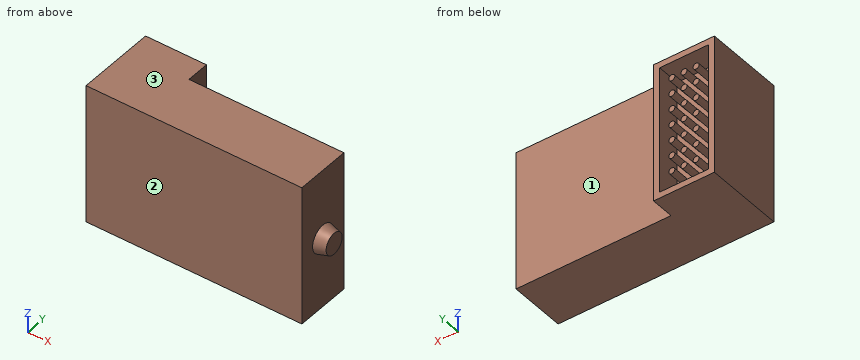
```python
from build123d import *

# Parameters (mm, degrees)
SKETCH1_W           = 35.5
SKETCH1_H           = 23
BOSS_EXTRUDE1_DEPTH = 9.18
SKETCH2_W           = 10
SKETCH2_H           = 23
SKETCH2_W_2         = 8
SKETCH2_H_2         = 21
BOSS_EXTRUDE2_DEPTH = 3.82
SKETCH3_R           = 0.5
BOSS_EXTRUDE3_DEPTH = 3.82


with BuildPart() as part:
    # Sketch1 → Boss-Extrude1 (new body)
    with BuildSketch(Plane(origin=(0, 0, 0), x_dir=(1, 0, 0), z_dir=(0, 1, 0))):
        Rectangle(SKETCH1_W, SKETCH1_H)
    extrude(amount=BOSS_EXTRUDE1_DEPTH)

    # Sketch2 → Boss-Extrude2 (add)
    with BuildSketch(Plane(origin=(0, 9.18, 0), x_dir=(1, 0, 0), z_dir=(0, 1, 0))):
        with Locations((-12.75, 0)):
            Rectangle(SKETCH2_W, SKETCH2_H)
        with Locations((-12.75, 0)):
            Rectangle(SKETCH2_W_2, SKETCH2_H_2, mode=Mode.SUBTRACT)
    extrude(amount=BOSS_EXTRUDE2_DEPTH)

    # Sketch3 → Boss-Extrude3 (add)
    with BuildSketch(Plane(origin=(0, 9.18, 0), x_dir=(1, 0, 0), z_dir=(0, 1, 0))):
        with Locations(Location((-14.75, 7.875, 0), (0, 0, 90))):
            Circle(SKETCH3_R)
        with Locations(Location((-12.75, 7.875, 0), (0, 0, 90))):
            Circle(SKETCH3_R)
        with Locations(Location((-10.75, 7.875, 0), (0, 0, 90))):
            Circle(SKETCH3_R)
        with Locations(Location((-12.75, 5.25, 0), (0, 0, 90))):
            Circle(SKETCH3_R)
        with Locations(Location((-10.75, 5.25, 0), (0, 0, 90))):
            Circle(SKETCH3_R)
        with Locations(Location((-12.75, 2.625, 0), (0, 0, 90))):
            Circle(SKETCH3_R)
        with Locations(Location((-10.75, 2.625, 0), (0, 0, 90))):
            Circle(SKETCH3_R)
        with Locations(Location((-12.75, 0, 0), (0, 0, 90))):
            Circle(SKETCH3_R)
        with Locations(Location((-10.75, 0, 0), (0, 0, 90))):
            Circle(SKETCH3_R)
        with Locations(Location((-12.75, -2.625, 0), (0, 0, 90))):
            Circle(SKETCH3_R)
        with Locations(Location((-10.75, -2.625, 0), (0, 0, 90))):
            Circle(SKETCH3_R)
        with Locations(Location((-12.75, -5.25, 0), (0, 0, 90))):
            Circle(SKETCH3_R)
        with Locations(Location((-10.75, -5.25, 0), (0, 0, 90))):
            Circle(SKETCH3_R)
        with Locations(Location((-12.75, -7.875, 0), (0, 0, 90))):
            Circle(SKETCH3_R)
        with Locations(Location((-10.75, -7.875, 0), (0, 0, 90))):
            Circle(SKETCH3_R)
        with Locations(Location((-14.75, 5.25, 0), (0, 0, 90))):
            Circle(SKETCH3_R)
        with Locations(Location((-14.75, 2.625, 0), (0, 0, 90))):
            Circle(SKETCH3_R)
        with Locations(Location((-14.75, 0, 0), (0, 0, 90))):
            Circle(SKETCH3_R)
        with Locations(Location((-14.75, -2.625, 0), (0, 0, 90))):
            Circle(SKETCH3_R)
        with Locations(Location((-14.75, -5.25, 0), (0, 0, 90))):
            Circle(SKETCH3_R)
        with Locations(Location((-14.75, -7.875, 0), (0, 0, 90))):
            Circle(SKETCH3_R)
    extrude(amount=BOSS_EXTRUDE3_DEPTH)

    # Sketch5 → Revolve1 (revolve)
    with BuildSketch(Plane.XY, mode=Mode.PRIVATE) as revolve1_sk:
        Polygon((17.75, 4.59), (19.6, 4.59), (19.6, 6.34), (17.75, 6.84), align=None)
    revolve(revolve1_sk.sketch.rotate(Axis((17.75, 4.59, 0), (1, 0, 0)), 90), axis=Axis((17.75, 4.59, 0), (1, 0, 0)))


solid = part.part
```
Read the model definition and answer for the solid it produces. Units are mm, in the model's axes. Face numbers are marked on the shaded views. Coordinates: 2 decimals unless noted, no trailing zeros. Write each loop counter-clockwise with the first axis right and the second up, starting at its lowest first coordinate (ties: lowest second). Pieces come first, ordered by that corner, then holes. Notation, with made-up numbers: (1, 6.25) - (26, 6.25) arc R31 ccw to (26, 35.25) - close; hole circle Ø11 at (-22.5, -6). An arc over 180 degrees is marked (long way). Answer as a JSON object with one key per item and string values. Group by question number.
1. A cutting plane is placed at C-C (y = 4.59). Determine the outline of the cut face in (x, z).
2. The mould has two halves that part along Y. Classify the marked faces 1, 2 and 3: +Y half, -Y half, draft (parallel to the pull), parting line (faces both ways), or undercut.
3. Consider L1, parallel to X at y = 9.25, z = 6.5; L2, parallel to Y at x = 5.5, z = 9.25; L3, parallel to Z at x = -14, y = 11.25. Determine where each line is inside the solid, lowest interval first. Write a range as [from, to].
4. A cutting plane is placed at A-A (y = 10). Give the number of separate pieces and of enclosed holes in the cut face, plus the area to 3 significant figures.
5. Each of these flat-tipped pins is pushed along its axis until it touches: P1, Ø6, axis at y = 9.5, z = 4, coming from the +X side; P2, Ø3, axis at y = 11.5, z = 3.5, coming from the +X side; P3, Ø5, axis at x = 10.5, y = 10, coming from the +Z side; P4, Ø7, axis at x = -1, z = -5.5, coming from the +Y side. Where does it stop, or does it pass through?
6. A cutting plane is placed at B-B (z = -5.25). Determine the outline of the cut face in (x, y), plus the area to 3 significant figures.
7. A cutting plane is placed at D-D (z = 0). Determine the outline of the cut face in (x, y), plus the area to 3 significant figures.
Worked out:
{
 "1": {"outline": "(-17.75, -11.5) - (17.75, -11.5) - (17.75, -2.25) - (19.6, -1.75) - (19.6, 1.75) - (17.75, 2.25) - (17.75, 11.5) - (-17.75, 11.5) - close"},
 "2": {"face 1": "+Y half", "face 2": "-Y half", "face 3": "draft"},
 "3": {"L1": "x = [-17.75, -16.75], [-8.75, -7.75]", "L2": "y = [0, 9.18]", "L3": "z = [-11.5, -10.5], [10.5, 11.5]"},
 "4": {"separate pieces": "22", "enclosed holes": "1", "area": "78.5 mm²"},
 "5": {"P1": "stops at x = 17.75", "P2": "stops at x = -7.75", "P3": "stops at z = 11.5", "P4": "stops at y = 9.18"},
 "6": {"outline": "(-17.75, 0) - (17.75, 0) - (17.75, 9.18) - (-7.75, 9.18) - (-7.75, 13) - (-8.75, 13) - (-8.75, 9.18) - (-10.25, 9.18) - (-10.25, 13) - (-11.25, 13) - (-11.25, 9.18) - (-12.25, 9.18) - (-12.25, 13) - (-13.25, 13) - (-13.25, 9.18) - (-14.25, 9.18) - (-14.25, 13) - (-15.25, 13) - (-15.25, 9.18) - (-16.75, 9.18) - (-16.75, 13) - (-17.75, 13) - close", "area": "345 mm²"},
 "7": {"outline": "(-17.75, 0) - (17.75, 0) - (17.75, 2.34) - (19.6, 2.84) - (19.6, 6.34) - (17.75, 6.84) - (17.75, 9.18) - (-7.75, 9.18) - (-7.75, 13) - (-8.75, 13) - (-8.75, 9.18) - (-10.25, 9.18) - (-10.25, 13) - (-11.25, 13) - (-11.25, 9.18) - (-12.25, 9.18) - (-12.25, 13) - (-13.25, 13) - (-13.25, 9.18) - (-14.25, 9.18) - (-14.25, 13) - (-15.25, 13) - (-15.25, 9.18) - (-16.75, 9.18) - (-16.75, 13) - (-17.75, 13) - close", "area": "352 mm²"}
}
